The listing builds one solid part. Answer for the finished solid, in the listing's coordinates (mm). Face numbers are marked on the shaded views. A direction names the side the tool comes from. Give positions to 0.01 mm unless a question says otherwise; leave off trailing zeros. Write each loop counter-clockwise with the first axis right and the second up, starting at its lowest first coordinate (ties: lowest second). Pieces come first, ordered by that corner, then holes. Notation, with made-up numbers: (-34.5, 56) - (12.5, 56) arc R24 ccw to (12.5, 80) - close; hole circle Ø4 at (-5, -31). An arc over 180 degrees is marked (long way). Write each question's results on one line, items separated by ' | '. Start each with the question number.
Q1. Find the intervals of material crossed by probe 1 along X at (y, z) = (2, 2.75); probe 2 along Y at (x, z) = (29, 1.7); probe 3 along Y at (x, z) = (9, 3.1) (3 decimals), in increasing order.
Q2. Flat-ended cylindrical pins translate along their axes: pin 1 Ø1 at (x, z) = (28, 3.5) entering from +Y; pin 2 Ø2.5 at (x, z) = (18.5, 3.5) entering from -Y (3 decimals). Find the tip coordinate at first contact, or state that the pin passes through.
Q3. For the marked faces 1, 2 and 3, determine the directions among +Z, -Z, +X, -X, +Y, -Y from which every point of the face is accessible in a straight line to the end or side of a thin tool.
Q4. For a pull along X with two mould halves and no side action, classify the marked faces 4, 5 and 6 as pulls with the +X half, pulls with the -X half, needs draft (parallel to the pull), parting line crosses it, or undercut.
Q5. Section B-B (y = 35) is taken. Determine the outline of the cut face in (x, z).
Q6. Section C-C (z = 1.45) is taken. State how many separate pieces and enclosed holes the cut face has, plus the area to 3 significant figures.
Q7. Section A-A (y = 8.5) is taken. Determine the outline of the cut face in (x, z), plus the area to 3 significant figures.
Q8. Section D-D (x = 10.5) is taken. Determine the outline of the cut face in (y, z) (3 decimals).
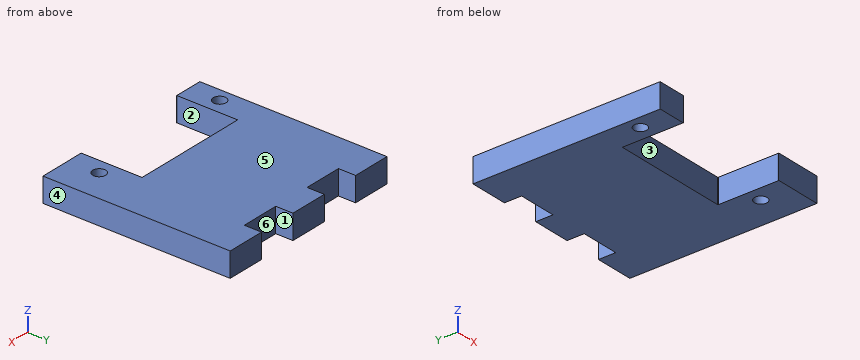
```python
from build123d import *

# Parameters (mm, degrees)
SKETCH1_W           = 38.1
SKETCH1_H           = 37.084
BOSS_EXTRUDE1_DEPTH = 4.826
SKETCH3_R           = 1.27
CUT_EXTRUDE2_DEPTH  = 54.386546358
CUT_EXTRUDE3_DEPTH  = 54.386546358
SKETCH5_W           = 7.62
SKETCH5_H           = 3.409901171
CUT_EXTRUDE4_DEPTH  = 54.386546358


with BuildPart() as part:
    # Sketch1 → Boss-Extrude1 (new body)
    with BuildSketch(Plane.XY):
        with Locations((19.05, 18.542)):
            Rectangle(SKETCH1_W, SKETCH1_H)
    extrude(amount=BOSS_EXTRUDE1_DEPTH)

    # Sketch3 → Cut-Extrude2 (cut, through all)
    with BuildSketch(Plane.XY.offset(4.826)):
        with Locations((2.580480538, 6.0325)):
            Circle(SKETCH3_R)
        with Locations((31.836519462, 6.0325)):
            Circle(SKETCH3_R)
    extrude(amount=-CUT_EXTRUDE2_DEPTH, mode=Mode.SUBTRACT)

    # Sketch4 → Cut-Extrude3 (cut, through all)
    with BuildSketch(Plane(origin=(0, 0, 0), x_dir=(-1, 0, 0), z_dir=(0, 0, -1))):
        with BuildLine():
            Line((-28.702, 12.065), (-5.715, 12.065))
            ThreePointArc((-5.715, 12.065), (-5.625197439, 12.027802561), (-5.588, 11.938))
            Line((-5.588, 11.938), (-5.588, 0.127))
            ThreePointArc((-5.588, 0.127), (-5.625197439, 0.037197439), (-5.715, 0))
            Line((-5.715, 0), (-28.702, 0))
            ThreePointArc((-28.702, 0), (-28.791802561, 0.037197439), (-28.829, 0.127))
            Line((-28.829, 0.127), (-28.829, 11.938))
            ThreePointArc((-28.829, 11.938), (-28.791802561, 12.027802561), (-28.702, 12.065))
        make_face()
    extrude(amount=-CUT_EXTRUDE3_DEPTH, mode=Mode.SUBTRACT)

    # Sketch5 → Cut-Extrude4 (cut, through all)
    with BuildSketch(Plane.XY.offset(4.826)):
        with Locations((11.43, 35.379049415)):
            Rectangle(SKETCH5_W, SKETCH5_H)
        with Locations((26.67, 35.379049415)):
            Rectangle(SKETCH5_W, SKETCH5_H)
    extrude(amount=-CUT_EXTRUDE4_DEPTH, mode=Mode.SUBTRACT)


solid = part.part
```
Answers below:
1) probe 1: x = 0 to 5.59, 28.83 to 38.1 | probe 2: y = 0 to 33.67 | probe 3: y = 12.065 to 33.674
2) pin 1: stops at y = 33.67 | pin 2: stops at y = 12.065
3) face 1: +Z, -Z, +Y | face 2: +Z, -Z | face 3: +Z, -Z, -Y
4) face 4: pulls with the +X half | face 5: needs draft | face 6: undercut
5) outline: (0, 0) - (7.62, 0) - (7.62, 4.83) - (0, 4.83) - close; (15.24, 0) - (22.86, 0) - (22.86, 4.83) - (15.24, 4.83) - close; (30.48, 0) - (38.1, 0) - (38.1, 4.83) - (30.48, 4.83) - close
6) separate pieces: 1 | enclosed holes: 2 | area: 1,070 mm2
7) outline: (0, 0) - (5.59, 0) - (5.59, 4.83) - (0, 4.83) - close; (28.83, 0) - (38.1, 0) - (38.1, 4.83) - (28.83, 4.83) - close | area: 71.7 mm2
8) outline: (12.065, 0) - (33.674, 0) - (33.674, 4.826) - (12.065, 4.826) - close
